Verification items for this drawing (mm, ordinates from the low corner). A direction names the side the tool comes from. Round coordinates to 2 decimals unless told otherwise and drop trailing zeros. Loops run counter-clockwise (first coordinate to the right, second up) from the corner with the lowest first, then second, coordinate; pieces in that order, holes last. Notation, with made-up numbers: (12.25, 87) - (27.25, 87) arc R17 ccw to (27.25, 115) - close; hole circle Ø10 at (-30.5, 15.25). An arc over 180 degrees is marked (long way). Answer in a Markdown table with one row per item. Add a question column.
(1) Cross-section at B-B on z = 4.5. Enter the section's corners in (x, y).
(2) Cross-section at D-D on y = 3.25. Enter the section's corners in (x, z), then the cut area to 3 significant figures.
(3) Cross-section at A-A on x = 8.5. Enter the section's corners in (y, z).
(4) Mould release check, pull along X, two halves, no side actions. Record for the marked faces 1, 2, 3 and 4: +X half, -X half, draft (parallel to the pull), parting line (faces both ways), or undercut.
(5) Access from +Z, -Z, +X, -X, +Y, -Y to the whole of each face (thin tool, end or side, straight path). Record for the marked faces 5, 6 and 7.
(6) Gauge pin test, flat ends, axial feed: pin 1 (1 mm diameter, centred on x = 9, z = 12, fed in from +Y); pin 2 (0.6 mm diameter, centred on x = 8.5, z = 12, fed in from -Y); pin 3 (2 mm diameter, centred on x = 2, z = 11, fed in from +Y). Record the tip position at first contact, or that the pin passes through.
(7) Thickness scan on line 1 along Y through (x, z) = (8.5, 11.55); line 2 along X through (y, z) = (2, 7.5); line 3 along Z through (x, y) = (7.25, 9). Record the ranges inside material, lowest first.
(8) Cross-section at C-C on y = 4.75. Enter the section's corners in (x, z).
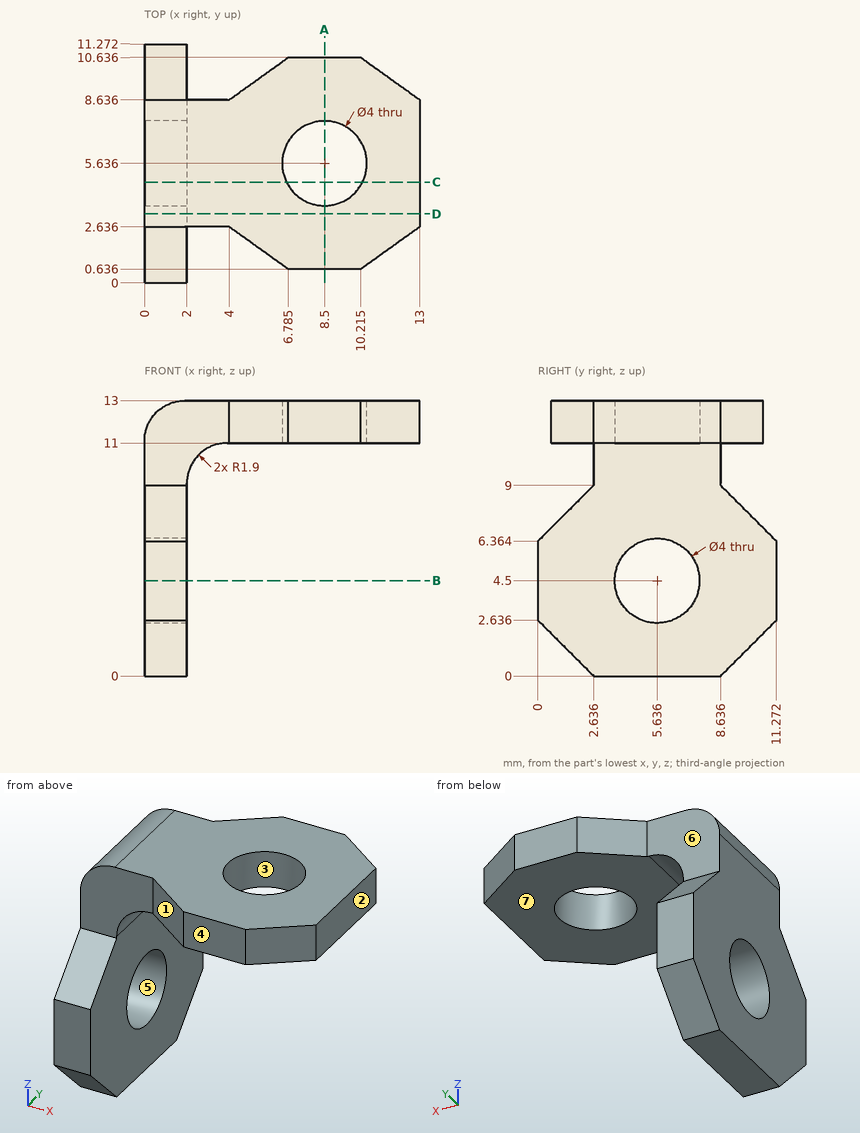
Answers:
| question | item | result |
|---|---|---|
| 1 | outline | (0, 0) - (2, 0) - (2, 3.64) - (0, 3.64) - close; (0, 7.64) - (2, 7.64) - (2, 11.27) - (0, 11.27) - close |
| 2 | outline | (0, 0) - (2, 0) - (2, 9.1) arc R1.9 cw to (3.9, 11) - (13, 11) - (13, 13) - (1.9, 13) arc R1.9 ccw to (0, 11.1) - close |
| 2 | area | 48.0 mm^2 |
| 3 | outline | (0.64, 11) - (3.64, 11) - (3.64, 13) - (0.64, 13) - close; (7.64, 11) - (10.64, 11) - (10.64, 13) - (7.64, 13) - close |
| 4 | face 1 | -X half |
| 4 | face 2 | +X half |
| 4 | face 3 | undercut |
| 4 | face 4 | draft |
| 5 | face 5 | +X, -X |
| 5 | face 6 | +Z, -X, +Y |
| 5 | face 7 | -Z, +X, +Y, -Y |
| 6 | pin 1 | stops at y = 10.64 |
| 6 | pin 2 | stops at y = 0.64 |
| 6 | pin 3 | stops at y = 8.64 |
| 7 | line 1 | y = 0.64 to 3.64, 7.64 to 10.64 |
| 7 | line 2 | x = 0 to 2 |
| 7 | line 3 | z = 11 to 13 |
| 8 | outline | (0, 0) - (2, 0) - (2, 2.71) - (0, 2.71) - close; (0, 6.29) - (2, 6.29) - (2, 9.1) arc R1.9 cw to (3.9, 11) - (6.71, 11) - (6.71, 13) - (1.9, 13) arc R1.9 ccw to (0, 11.1) - close; (10.29, 11) - (13, 11) - (13, 13) - (10.29, 13) - close |
